Part model, mm, in its own coordinate system. Round coordinates to 2 decimals unless told otherwise and drop trailing zeros. Write each loop counter-clockwise with the first axis right and the second up, starting at its lowest first coordinate (ties: lowest second). Pieces come first, ordered by that corner, then holes. Notation, with made-up numbers: M 73,52 L 124,52 A14 cw 124,61 Z; hole C 88.5,74 d10. An arc over 180 degrees is marked long. Use one line per item in the form item = value. Start each with the question number.
Item 1: Cut at B-B, the plane x = 84. Give the cut face in (y, z).
Item 2: Probe L1, parallel to X at y = -74, z = 0.45; L2, parallel to Y at x = -39, z = 1.35; L3, parallel to Y at x = -94.5, z = 0.2. List the from-to ranges inside material, lowest first.
Item 3: Cut at A-A, the plane x = 0. State how many separate pieces and enclosed holes the cut face has, then the cut area to 3 significant figures.
Item 4: Mould opens along X. For faces 1 (the face through (-59.427, 0.398, 0.749)), 2 (the face through (100.15, 31.54, 0.75)), 3 (the face through (75.8, -43.87, 0.75)) say: +X half, -X half, draft (parallel to the pull), parting line (faces both ways), or undercut.
from build123d import *

# Parameters (mm, degrees)
F0_R     = 105
F0_R_2   = 9.525
F0_R_3   = 2.38125
F1_DEPTH = 1.51892


with BuildPart() as f1:
    # F0 (on Top) → F1 (new body)
    with BuildSketch(Plane.XY):
        Circle(F0_R)
        with Locations((-69.270038, -59.997693)):
            Circle(F0_R_2, mode=Mode.SUBTRACT)
        with Locations((-25.817276, -87.929117)):
            Circle(F0_R_2, mode=Mode.SUBTRACT)
        with Locations((-49.561652, -77.082449)):
            Circle(F0_R_2, mode=Mode.SUBTRACT)
        with Locations((-30.518334, -62.830357)):
            Circle(F0_R_2, mode=Mode.SUBTRACT)
        with Locations((-0.274165, -69.849462)):
            Circle(F0_R_2, mode=Mode.SUBTRACT)
        with Locations((-83.367003, -38.05265)):
            Circle(F0_R_2, mode=Mode.SUBTRACT)
        with Locations((-54.732814, -43.397483)):
            Circle(F0_R_2, mode=Mode.SUBTRACT)
        with Locations((-90.710582, -13.025041)):
            Circle(F0_R_2, mode=Mode.SUBTRACT)
        with Locations((-68.133405, -15.39031)):
            Circle(F0_R_2, mode=Mode.SUBTRACT)
        with Locations((-40.369083, -29.350384)):
            Circle(F0_R_2, mode=Mode.SUBTRACT)
        with Locations((-15.4115, -47.472029)):
            Circle(F0_R_2, mode=Mode.SUBTRACT)
        with Locations((-49.910996, -0.02076)):
            Circle(F0_R_2, mode=Mode.SUBTRACT)
        with Locations((-20.364587, -20.364587)):
            Circle(F0_R_2, mode=Mode.SUBTRACT)
        with Locations((0, -91.640937)):
            Circle(F0_R_2, mode=Mode.SUBTRACT)
        with Locations((25.817276, -87.929117)):
            Circle(F0_R_2, mode=Mode.SUBTRACT)
        with Locations((49.543149, -77.094343)):
            Circle(F0_R_2, mode=Mode.SUBTRACT)
        with Locations((30.518334, -62.830357)):
            Circle(F0_R_2, mode=Mode.SUBTRACT)
        with Locations((69.255635, -60.014318)):
            Circle(F0_R_2, mode=Mode.SUBTRACT)
        with Locations((15.431245, -47.465615)):
            Circle(F0_R_2, mode=Mode.SUBTRACT)
        with Locations((0, -28.799874)):
            Circle(F0_R_2, mode=Mode.SUBTRACT)
        with Locations((40.381288, -29.333591)):
            Circle(F0_R_2, mode=Mode.SUBTRACT)
        with Locations((20.364587, -20.364587)):
            Circle(F0_R_2, mode=Mode.SUBTRACT)
        with Locations((54.732814, -43.397483)):
            Circle(F0_R_2, mode=Mode.SUBTRACT)
        with Locations((83.357867, -38.072659)):
            Circle(F0_R_2, mode=Mode.SUBTRACT)
        with Locations((68.133405, -15.39031)):
            Circle(F0_R_2, mode=Mode.SUBTRACT)
        with Locations((90.707453, -13.046813)):
            Circle(F0_R_2, mode=Mode.SUBTRACT)
        with Locations((-90.705887, 13.057699)):
            Circle(F0_R_2, mode=Mode.SUBTRACT)
        with Locations((-68.072472, 15.657619)):
            Circle(F0_R_2, mode=Mode.SUBTRACT)
        with Locations((-83.353297, 38.082663)):
            Circle(F0_R_2, mode=Mode.SUBTRACT)
        with Locations((-54.562055, 43.611979)):
            Circle(F0_R_2, mode=Mode.SUBTRACT)
        with Locations((-28.799874, 0)):
            Circle(F0_R_2, mode=Mode.SUBTRACT)
        with Locations((-20.364587, 20.364587)):
            Circle(F0_R_2, mode=Mode.SUBTRACT)
        with Locations((-40.393485, 29.316792)):
            Circle(F0_R_2, mode=Mode.SUBTRACT)
        with Locations((-15.450986, 47.459192)):
            Circle(F0_R_2, mode=Mode.SUBTRACT)
        with Locations((-69.248432, 60.022629)):
            Circle(F0_R_2, mode=Mode.SUBTRACT)
        with Locations((-30.271487, 62.949659)):
            Circle(F0_R_2, mode=Mode.SUBTRACT)
        with Locations((-49.533896, 77.100289)):
            Circle(F0_R_2, mode=Mode.SUBTRACT)
        with Locations((-25.806723, 87.932215)):
            Circle(F0_R_2, mode=Mode.SUBTRACT)
        Circle(F0_R_3, mode=Mode.SUBTRACT)
        with Locations((20.364587, 20.364587)):
            Circle(F0_R_2, mode=Mode.SUBTRACT)
        with Locations((28.799874, 0)):
            Circle(F0_R_2, mode=Mode.SUBTRACT)
        with Locations((49.911, 0)):
            Circle(F0_R_2, mode=Mode.SUBTRACT)
        with Locations((0, 28.799874)):
            Circle(F0_R_2, mode=Mode.SUBTRACT)
        with Locations((15.431245, 47.465615)):
            Circle(F0_R_2, mode=Mode.SUBTRACT)
        with Locations((40.381288, 29.333591)):
            Circle(F0_R_2, mode=Mode.SUBTRACT)
        with Locations((68.072472, 15.657619)):
            Circle(F0_R_2, mode=Mode.SUBTRACT)
        with Locations((90.709018, 13.035927)):
            Circle(F0_R_2, mode=Mode.SUBTRACT)
        with Locations((54.562055, 43.611979)):
            Circle(F0_R_2, mode=Mode.SUBTRACT)
        with Locations((83.362436, 38.062655)):
            Circle(F0_R_2, mode=Mode.SUBTRACT)
        with Locations((0, 69.85)):
            Circle(F0_R_2, mode=Mode.SUBTRACT)
        with Locations((30.271487, 62.949659)):
            Circle(F0_R_2, mode=Mode.SUBTRACT)
        with Locations((49.552401, 77.088397)):
            Circle(F0_R_2, mode=Mode.SUBTRACT)
        with Locations((0.010998, 91.640937)):
            Circle(F0_R_2, mode=Mode.SUBTRACT)
        with Locations((25.827829, 87.926018)):
            Circle(F0_R_2, mode=Mode.SUBTRACT)
        with Locations((69.262837, 60.006006)):
            Circle(F0_R_2, mode=Mode.SUBTRACT)
    extrude(amount=F1_DEPTH)


solid = f1.part
Model answer:
q1.outline = M -63,0 L -47.58,0 L -47.58,1.52 L -63,1.52 Z; M -28.57,0 L -19.81,0 L -19.81,1.52 L -28.57,1.52 Z; M -6.28,0 L 6.27,0 L 6.27,1.52 L -6.28,1.52 Z; M 19.8,0 L 28.56,0 L 28.56,1.52 L 19.8,1.52 Z; M 47.57,0 L 63,0 L 63,1.52 L 47.57,1.52 Z
q2.L1 = -74.49 to -58.57, -40.55 to -8.85, 8.3 to 40.53, 58.55 to 74.49
q2.L2 = -97.49 to -67.16, -58.5 to -38.78, -19.92 to 19.89, 38.74 to 59.14, 66.76 to 97.49
q2.L3 = -45.77 to -21.76, -4.29 to 4.32, 21.79 to 45.77
q3.separate_pieces = 8
q3.enclosed_holes = 0
q3.area = 138 mm²
q4.face_1 = undercut
q4.face_2 = parting line
q4.face_3 = undercut
